from build123d import *

# Parameters (mm, degrees)
F1_DEPTH  = 4
F3_DEPTH  = 4
F4_R      = 1.5
F5_DEPTH  = 25
F6_R      = 1.5
F7_DEPTH  = 25
F8_R      = 1.5
F9_DEPTH  = 25
F10_R     = 1.5
F11_DEPTH = 5


with BuildPart() as f1:
    # F0 (on Top) → F1 (new body)
    with BuildSketch(Plane.XY):
        Polygon((40, 107.510013), (0, 107.510013), (-40, 107.510013), (-60, 98.002009), (-60, 71.096797), (-45, 62.30734), (-45, -32.69266), (-60, -38.903203), (-60, -62.073313), (-36.951705, -76.219407), (0, -76.219407), (36.951705, -76.219407), (60, -62.073313), (60, -38.903203), (45, -32.69266), (45, 62.30734), (60, 71.096797), (60, 98.002009), align=None)
        with BuildLine():
            Line((-14.5, -44.219407), (0, -44.219407))
            Line((0, -44.219407), (14.5, -44.219407))
            ThreePointArc((14.5, -44.219407), (16.62132, -45.098087), (17.5, -47.219407))
            Line((17.5, -47.219407), (17.5, -58.219407))
            ThreePointArc((17.5, -58.219407), (16.62132, -60.340728), (14.5, -61.219407))
            Line((14.5, -61.219407), (0, -61.219407))
            Line((0, -61.219407), (-14.5, -61.219407))
            ThreePointArc((-14.5, -61.219407), (-16.62132, -60.340728), (-17.5, -58.219407))
            Line((-17.5, -58.219407), (-17.5, -47.219407))
            ThreePointArc((-17.5, -47.219407), (-16.62132, -45.098087), (-14.5, -44.219407))
        make_face(mode=Mode.SUBTRACT)
        with BuildLine():
            Line((-14.5, 97.510013), (0, 97.510013))
            Line((0, 97.510013), (14.5, 97.510013))
            ThreePointArc((14.5, 97.510013), (16.62132, 96.631334), (17.5, 94.510013))
            Line((17.5, 94.510013), (17.5, 83.510013))
            ThreePointArc((17.5, 83.510013), (16.62132, 81.388693), (14.5, 80.510013))
            Line((14.5, 80.510013), (0, 80.510013))
            Line((0, 80.510013), (-14.5, 80.510013))
            ThreePointArc((-14.5, 80.510013), (-16.62132, 81.388693), (-17.5, 83.510013))
            Line((-17.5, 83.510013), (-17.5, 94.510013))
            ThreePointArc((-17.5, 94.510013), (-16.62132, 96.631334), (-14.5, 97.510013))
        make_face(mode=Mode.SUBTRACT)
    extrude(amount=F1_DEPTH)

    # F2 (on face) → F3 (join)
    with BuildSketch(Plane(origin=(0, 0, 0), x_dir=(1, 0, 0), z_dir=(0, 0, -1))):
        with BuildLine():
            Line((15.5, 68.219407), (-15.5, 68.219407))
            ThreePointArc((-15.5, 68.219407), (-16.914214, 67.633621), (-17.5, 66.219407))
            Line((-17.5, 66.219407), (-17.5, 63.219407))
            ThreePointArc((-17.5, 63.219407), (-16.914214, 61.805194), (-15.5, 61.219407))
            Line((-15.5, 61.219407), (15.5, 61.219407))
            ThreePointArc((15.5, 61.219407), (16.914214, 61.805194), (17.5, 63.219407))
            Line((17.5, 63.219407), (17.5, 66.219407))
            ThreePointArc((17.5, 66.219407), (16.914214, 67.633621), (15.5, 68.219407))
        make_face()
        with BuildLine():
            Line((15.5, 44.219407), (-15.5, 44.219407))
            ThreePointArc((-15.5, 44.219407), (-16.914214, 43.633621), (-17.5, 42.219407))
            Line((-17.5, 42.219407), (-17.5, 39.219407))
            ThreePointArc((-17.5, 39.219407), (-16.914214, 37.805194), (-15.5, 37.219407))
            Line((-15.5, 37.219407), (15.5, 37.219407))
            ThreePointArc((15.5, 37.219407), (16.914214, 37.805194), (17.5, 39.219407))
            Line((17.5, 39.219407), (17.5, 42.219407))
            ThreePointArc((17.5, 42.219407), (16.914214, 43.633621), (15.5, 44.219407))
        make_face()
        with BuildLine():
            Line((15.5, -73.510013), (-15.5, -73.510013))
            ThreePointArc((-15.5, -73.510013), (-16.914214, -74.0958), (-17.5, -75.510013))
            Line((-17.5, -75.510013), (-17.5, -78.510013))
            ThreePointArc((-17.5, -78.510013), (-16.914214, -79.924227), (-15.5, -80.510013))
            Line((-15.5, -80.510013), (15.5, -80.510013))
            ThreePointArc((15.5, -80.510013), (16.914214, -79.924227), (17.5, -78.510013))
            Line((17.5, -78.510013), (17.5, -75.510013))
            ThreePointArc((17.5, -75.510013), (16.914214, -74.0958), (15.5, -73.510013))
        make_face()
        with BuildLine():
            Line((15.5, -97.510013), (-15.5, -97.510013))
            ThreePointArc((-15.5, -97.510013), (-16.914214, -98.0958), (-17.5, -99.510013))
            Line((-17.5, -99.510013), (-17.5, -102.510013))
            ThreePointArc((-17.5, -102.510013), (-16.914214, -103.924227), (-15.5, -104.510013))
            Line((-15.5, -104.510013), (15.5, -104.510013))
            ThreePointArc((15.5, -104.510013), (16.914214, -103.924227), (17.5, -102.510013))
            Line((17.5, -102.510013), (17.5, -99.510013))
            ThreePointArc((17.5, -99.510013), (16.914214, -98.0958), (15.5, -97.510013))
        make_face()
    extrude(amount=F3_DEPTH)

    # F4 (on face) → F5 (cut)
    with BuildSketch(Plane.XY.offset(4)):
        with Locations((-20.5, 48.30734)):
            Circle(F4_R)
        with Locations((-20.5, -3.69266)):
            Circle(F4_R)
        with Locations((20.5, 48.30734)):
            Circle(F4_R)
        with Locations((20.5, -3.69266)):
            Circle(F4_R)
    extrude(amount=-F5_DEPTH, mode=Mode.SUBTRACT)

    # F6 (on face) → F7 (cut)
    with BuildSketch(Plane.XY.offset(4)):
        with Locations((-13, -40.219407)):
            Circle(F6_R)
        with Locations((-13, -65.219407)):
            Circle(F6_R)
        with Locations((13, -40.219407)):
            Circle(F6_R)
        with Locations((13, -65.219407)):
            Circle(F6_R)
        with Locations((-13, 101.510013)):
            Circle(F6_R)
        with Locations((-13, 76.510013)):
            Circle(F6_R)
        with Locations((13, 101.510013)):
            Circle(F6_R)
        with Locations((13, 76.510013)):
            Circle(F6_R)
    extrude(amount=-F7_DEPTH, mode=Mode.SUBTRACT)

    # F8 (on face) → F9 (cut)
    with BuildSketch(Plane.XY.offset(4)):
        with Locations((-15, -2.383515)):
            Circle(F8_R)
        with Locations((-15, -27.383515)):
            Circle(F8_R)
        with Locations((15, -2.383515)):
            Circle(F8_R)
        with Locations((15, -27.383515)):
            Circle(F8_R)
        with Locations((-15, 64.966045)):
            Circle(F8_R)
        with Locations((-15, 39.966045)):
            Circle(F8_R)
        with Locations((15, 64.966045)):
            Circle(F8_R)
        with Locations((15, 39.966045)):
            Circle(F8_R)
        with Locations((0, 52.466045)):
            Circle(F8_R)
        with Locations((0, -14.883515)):
            Circle(F8_R)
    extrude(amount=-F9_DEPTH, mode=Mode.SUBTRACT)

    # F10 (on face) → F11 (join)
    with BuildSketch(Plane(origin=(0, 0, 0), x_dir=(1, 0, 0), z_dir=(0, 0, -1))):
        with BuildLine():
            Line((21.353659, -44.913041), (2.073171, -40.064042))
            ThreePointArc((2.073171, -40.064042), (0, -39.80734), (-2.073171, -40.064042))
            Line((-2.073171, -40.064042), (-21.353659, -44.913041))
            ThreePointArc((-21.353659, -44.913041), (-18.348001, -45.547104), (-17, -48.30734))
            ThreePointArc((-17, -48.30734), (-18.348001, -51.067576), (-21.353659, -51.70164))
            Line((-21.353659, -51.70164), (-2.073171, -56.550638))
            ThreePointArc((-2.073171, -56.550638), (0, -56.80734), (2.073171, -56.550638))
            Line((2.073171, -56.550638), (21.353659, -51.70164))
            ThreePointArc((21.353659, -51.70164), (17, -48.30734), (21.353659, -44.913041))
        make_face()
        with BuildLine():
            ThreePointArc((24, -48.30734), (23.260236, -46.155342), (21.353659, -44.913041))
            ThreePointArc((21.353659, -44.913041), (17, -48.30734), (21.353659, -51.70164))
            ThreePointArc((21.353659, -51.70164), (23.260236, -50.459339), (24, -48.30734))
        make_face()
        with Locations((20.5, -48.30734)):
            Circle(F10_R, mode=Mode.SUBTRACT)
        with BuildLine():
            ThreePointArc((-17, -48.30734), (-18.348001, -45.547104), (-21.353659, -44.913041))
            ThreePointArc((-21.353659, -44.913041), (-24, -48.30734), (-21.353659, -51.70164))
            ThreePointArc((-21.353659, -51.70164), (-18.348001, -51.067576), (-17, -48.30734))
        make_face()
        with Locations((-20.5, -48.30734)):
            Circle(F10_R, mode=Mode.SUBTRACT)
    extrude(amount=F11_DEPTH)


solid = f1.part
Read the model definition and answer for the solid it produces. Units are mm, in the model's axes. A direction names the side the tool comes from. Give positions to 0.01 mm unless a question says otherwise; leave off trailing zeros. Write each loop counter-clockwise with the first axis right and the second up, starting at its lowest first coordinate (ties: lowest second). Pieces come first, ordered by that corner, then holes. Notation, with made-up numbers: (-25, 56.5) - (9, 56.5) arc R36 ccw to (9, 95.5) - close; hole circle Ø6 at (61, 18). An arc over 180 degrees is marked (long way). Return JSON: item names as keys, results as strings.
Q1. A cutting plane is placed at B-B, the plane x = -28. Determine the outline of the cut face in (y, z), and give its area (3 significant figures).
Reply:
{"outline": "(-76.22, 0) - (107.51, 0) - (107.51, 4) - (-76.22, 4) - close", "area": "735 mm²"}
Q2. For faces 1 (the face through (-24, 48.2, -2.5)), 2 (the face through (45, 14, 2)), 3 (the face through (0, -68.219, -2)), 4 (the face through (17.5, -53, 2)), 5 (the face through (-0.029, 56.807, -2.465)), determine the directions among +Z, -Z, +X, -X, +Y, -Y from which every point of the face is accessible in a straight line to the end or side of a thin tool.
Reply:
{"face 1": "-Z, -X", "face 2": "+Z, -Z, +X", "face 3": "-Z, +X, -X, -Y", "face 4": "+Z, -Z", "face 5": "-Z"}
Q3. Consider line 1 along X through (y, z) = (-49.5, 3); line 2 along Y through (x, z) = (20.5, 2.15); line 3 along Y through (x, z) = (17, 0.25). Determine where each line is inside the solid, lowest interval first. Write a range as [from, to].
Reply:
{"line 1": "[-60, -17.5], [17.5, 60]", "line 2": "[-76.22, -5.19], [-2.19, 46.81], [49.81, 107.51]", "line 3": "[-76.22, -59.88], [-45.56, 81.85], [96.17, 107.51]"}
Q4. A cutting plane is placed at A-A, the plane y = 11. Determine the outline of the cut face in (x, z).
Reply:
{"outline": "(-45, 0) - (45, 0) - (45, 4) - (-45, 4) - close"}
Q5. Given P1, Ø2.5, axis at x = 3, z = -1, coming from the -Y side; P2, Ø2, axis at x = 1, z = -2.5, coming from the +Y side; P3, Ø1, axis at x = -29, y = -37, coming from the -Z side; P4, Ø2.5, axis at y = -64, z = -2.5, coming from the +X side, each flat-ended and moving along its own axis, determine where each tip first touches the part or whether it passes through.
Reply:
{"P1": "y = -76.22", "P2": "y = 104.51", "P3": "z = 0", "P4": "x = 17.5"}
Q6. A cutting plane is placed at C-C, the plane z = 2. Count the separate pieces of the cut face and the enclosed holes in it, and give its area (3 significant figures).
Reply:
{"separate pieces": "1", "enclosed holes": "24", "area": "17,100 mm²"}
Q7. For a pull along X with two mould halves and no side action, classify faces 6 (the face through (0, 97.51, 0)), 7 (the face through (-11.85, 54.09, -2.46)), 8 (the face through (50.14, 102.69, 1.97)) as released by +X, released by -X, zero draft, split by the parting line, or undercut.
Reply:
{"face 6": "undercut", "face 7": "released by -X", "face 8": "released by +X"}
